Here's how the part is built. I have some questions about the finished solid (model axes, mm). A direction names the side the tool comes from. Give positions to 0.01 mm unless a question says otherwise; leave off trailing zeros. Loops run counter-clockwise (first coordinate to the right, second up) from the corner with the lowest first, then second, coordinate; pieces in that order, holes last. Notation, with made-up numbers: (-14, 85.25) - (44, 85.25) arc R23 cw to (44, 107.25) - close; hole circle Ø9 at (78.5, 10). An arc over 180 degrees is marked (long way). Put each result on its own line as item: value. Start each with the question number.
from build123d import *

# Parameters (mm, degrees)
BOSS_EXTRUDE1_DEPTH = 1.59
SKETCH2_R           = 2.5
SKETCH2_R_2         = 1.75
CUT_EXTRUDE2_DEPTH  = 1.59
SKETCH3_W           = 1.59
SKETCH3_H           = 40
BOSS_EXTRUDE2_DEPTH = 30.602
SKETCH5_W           = 1.59
SKETCH5_H           = 40
CUT_EXTRUDE4_DEPTH  = 10
SKETCH9_W           = 30.602
SKETCH9_H           = 10
BOSS_EXTRUDE4_DEPTH = 1.59
SKETCH10_R          = 1.75
SKETCH10_R_2        = 2.5
CUT_EXTRUDE6_DEPTH  = 10
SKETCH11_R          = 1.25
CUT_EXTRUDE7_DEPTH  = 10


with BuildPart() as part:
    # Sketch1 → Boss-Extrude1 (new body)
    with BuildSketch(Plane.XY):
        with BuildLine():
            Line((-38.514035237, 20), (38.514035237, 20))
            ThreePointArc((38.514035237, 20), (58.514035237, 0), (38.514035237, -20))
            Line((38.514035237, -20), (-38.514035237, -20))
            Line((-38.514035237, -20), (-99.729964763, -20))
            Line((-99.729964763, -20), (-99.729964763, 20))
            Line((-99.729964763, 20), (-38.514035237, 20))
        make_face()
    extrude(amount=BOSS_EXTRUDE1_DEPTH)

    # Sketch2 → Cut-Extrude2 (cut)
    with BuildSketch(Plane.XY.offset(1.59)):
        with Locations((38.514035237, 0)):
            Circle(SKETCH2_R)
        with Locations((47.014035237, 0)):
            Circle(SKETCH2_R_2)
        with Locations((17.264035237, 0)):
            Circle(SKETCH2_R_2)
        with Locations((-12.735964763, 0)):
            Circle(SKETCH2_R_2)
        with Locations((-42.485964763, 0)):
            Circle(SKETCH2_R_2)
    extrude(amount=-CUT_EXTRUDE2_DEPTH, mode=Mode.SUBTRACT)

    # Sketch3 → Boss-Extrude2 (add)
    with BuildSketch(Plane.XY.offset(1.59)):
        with Locations((-98.934964763, 0)):
            Rectangle(SKETCH3_W, SKETCH3_H)
    extrude(amount=BOSS_EXTRUDE2_DEPTH)

    # Sketch5 → Cut-Extrude4 (cut)
    with BuildSketch(Plane.ZY.offset(99.729964763)):
        with Locations((31.397, 0)):
            Rectangle(SKETCH5_W, SKETCH5_H)
    extrude(amount=-CUT_EXTRUDE4_DEPTH, mode=Mode.SUBTRACT)

    # Sketch9 → Boss-Extrude4 (add)
    with BuildSketch(Plane.ZY.offset(99.729964763)):
        with Locations((15.301, 25)):
            Rectangle(SKETCH9_W, SKETCH9_H)
    extrude(amount=-BOSS_EXTRUDE4_DEPTH)

    # Sketch10 → Cut-Extrude6 (cut)
    with BuildSketch(Plane.ZY.offset(99.729964763)):
        with Locations((16.096, -8.5)):
            Circle(SKETCH10_R)
        with Locations((16.096, 0)):
            Circle(SKETCH10_R_2)
        with Locations((16.096, 21.25)):
            Circle(SKETCH10_R)
    extrude(amount=-CUT_EXTRUDE6_DEPTH, mode=Mode.SUBTRACT)

    # Sketch11 → Cut-Extrude7 (cut)
    with BuildSketch(Plane.XY.offset(1.59)):
        with Locations((-74.729964763, 0)):
            Circle(SKETCH11_R)
    extrude(amount=-CUT_EXTRUDE7_DEPTH, mode=Mode.SUBTRACT)


solid = part.part
1) Which directions (+Z, -Z, +X, -X, +Y, -Y) give clear straight access to the entire face, cutting with the end or side of a thin tool? Please do faces 4 (the cylindrical face through (-98.946, -7.974, 17.765)), 5 (the flat face through (-19, 0, 1.59)).
2) Suppose I cut it at A-A on y = -8.5. Please give me the cut outline in (x, z), plus the area to 3 significant figures.
3) Thinking about a two-plate mould opening in Y: for faces 1 (the flat face through (-30.9, -20, 0.5)), 2 (the cylindrical face through (58.51, 0.44, 0.78)), 3 (the cylindrical face through (-40.87, -0.67, 0.81)), which applies, pulls with the +Y half, pulls with the -Y half, needs draft (parallel to the pull), parting line crosses it, or undercut?
4) I'm going to push flat-ended pins straight in: P1, Ø4, axis at y = 8, z = 15.5, coming from the +X side; P2, Ø4, axis at y = -8.5, z = 16.096, coming from the -X side; P3, Ø4, axis at x = -42.49, y = 0, coming from the +Z side; P4, Ø0.8, axis at x = -44.5, z = 0.5, coming from the +Y side. Where does each tip first touch, or does it pass through?
5) Suppose I cut it at C-C on x = -86. Please give me the cut outline in (y, z), plus the area to 3 significant figures.
6) Suppose I cut it at B-B on z = 16. Please give me the cut outline in (x, y), plus the area to 3 significant figures.
7) Suppose I cut it at D-D on z = 24.5. Please give me the cut outline in (x, y), plus the area to 3 significant figures.
8) I need wall thicknesses on line 1 (X direction, y = -15, z = 29); line 2 (Z direction, x = -67.5, y = -1). Which ranges of each line are inside material? Lowest first, please.
Ans:
1. face 4: +X, -X
1. face 5: +Z, +X, +Y, -Y
2. outline: (-99.73, 0) - (56.62, 0) - (56.62, 1.59) - (-98.14, 1.59) - (-98.14, 14.35) - (-99.73, 14.35) - close; (-99.73, 17.85) - (-98.14, 17.85) - (-98.14, 30.6) - (-99.73, 30.6) - close
2. area: 289 mm²
3. face 1: pulls with the -Y half
3. face 2: parting line crosses it
3. face 3: undercut
4. P1: stops at x = -98.14
4. P2: stops at x = -99.73
4. P3: stops at z = 1.59
4. P4: stops at y = 20
5. outline: (-20, 0) - (20, 0) - (20, 1.59) - (-20, 1.59) - close
5. area: 63.6 mm²
6. outline: (-99.73, -20) - (-98.14, -20) - (-98.14, -10.25) - (-99.73, -10.25) - close; (-99.73, -6.75) - (-98.14, -6.75) - (-98.14, -2.5) - (-99.73, -2.5) - close; (-99.73, 2.5) - (-98.14, 2.5) - (-98.14, 19.5) - (-99.73, 19.5) - close; (-99.73, 23) - (-98.14, 23) - (-98.14, 30) - (-99.73, 30) - close
6. area: 60.4 mm²
7. outline: (-99.73, -20) - (-98.14, -20) - (-98.14, 30) - (-99.73, 30) - close
7. area: 79.5 mm²
8. line 1: x = -99.73 to -98.14
8. line 2: z = 0 to 1.59
